Read the model definition and answer for the solid it produces. Units are mm, in the model's axes. Coordinates: 2 decimals unless noted, no trailing zeros. Loops run counter-clockwise (first coordinate to the right, second up) from the corner with the lowest first, then second, coordinate; pieces in that order, holes last.
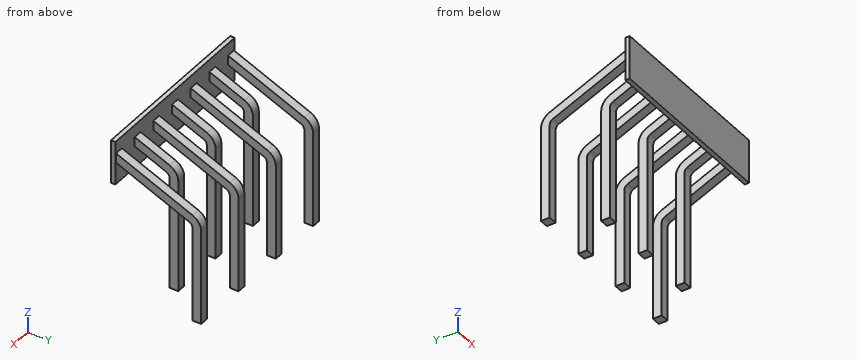
from build123d import *

# Parameters (mm, degrees)
SKETCH009_W            = 0.2
SKETCH009_H            = 2
PAD004_DEPTH           = 4.06
PAD005_DEPTH           = 0.2
LINEARPATTERN_COUNT    = 4
LINEARPATTERN_PITCH    = 2.54
PAD006_DEPTH           = 0.2
LINEARPATTERN001_COUNT = 3
LINEARPATTERN001_PITCH = 2.54


with BuildPart() as part:
    # Sketch009 (on DatumPlane) → Pad004 (new body, symmetric)
    with BuildSketch(Plane.YZ.offset(3.81)):
        with Locations((-3.8, 2.5)):
            Rectangle(SKETCH009_W, SKETCH009_H)
    extrude(amount=PAD004_DEPTH, both=True)

    # Sketch010 → Pad005 (join, symmetric)
    with BuildSketch(Plane.YZ):
        with BuildLine():
            Line((-0.2, -3.5), (-0.2, 0.85))
            ThreePointArc((-0.2, 0.85), (-0.241548, 0.988014), (-0.352383, 1.080154))
            Line((-0.352383, 1.080154), (-3.7, 2.5))
            Line((-3.7, 2.5), (-3.7, 2.934491))
            Line((-3.7, 2.934491), (-0.196196, 1.448401))
            ThreePointArc((0.2, 0.85), (0.091974, 1.208837), (-0.196196, 1.448401))
            Line((0.2, 0.85), (0.2, -3.5))
            Line((0.2, -3.5), (-0.2, -3.5))
        make_face()
    pad005 = extrude(amount=PAD005_DEPTH, both=True)

    # LinearPattern: Pad005 ×4
    with Locations(*[(i * LINEARPATTERN_PITCH, 0, 0) for i in range(1, LINEARPATTERN_COUNT)]):
        add(pad005)

    # Sketch011 (on DatumPlane) → Pad006 (join, symmetric)
    with BuildSketch(Plane.YZ.offset(1.27)):
        with BuildLine():
            Line((-3.7, 2.934491), (-3.7, 2.5))
            Line((-3.7, 2.5), (-2.257383, 1.888134))
            ThreePointArc((-2.105, 1.65798), (-2.146548, 1.795994), (-2.257383, 1.888134))
            Line((-2.105, 1.65798), (-2.105, -3.5))
            Line((-2.105, -3.5), (-1.705, -3.5))
            Line((-1.705, -3.5), (-1.705, 1.65798))
            ThreePointArc((-1.705, 1.65798), (-1.813026, 2.016816), (-2.101196, 2.256381))
            Line((-2.101196, 2.256381), (-3.7, 2.934491))
        make_face()
    pad006 = extrude(amount=PAD006_DEPTH, both=True)

    # LinearPattern001: Pad006 ×3
    with Locations(*[(i * LINEARPATTERN001_PITCH, 0, 0) for i in range(1, LINEARPATTERN001_COUNT)]):
        add(pad006)


solid = part.part
Q1. Flat-ended cylindrical pins translate along their axes: pin 1 Ø1 at (y, z) = (-2.5, 0) entering from +X; pin 2 Ø1.5 at (y, z) = (-2, 2.5) entering from -X; pin 3 Ø1.5 at (x, y) = (5.5, -3) entering from -Z. Find the tip coordinate at first contact, or state that the pin passes through.
Findings below:
pin 1: stops at x = 6.55
pin 2: stops at x = -0.2
pin 3: stops at z = 1.5
Q2. Straight lines are drawn through the part: probe 1 along X at (y, z) = (-2.05, -2.5); probe 2 along X at (y, z) = (0.05, -2.75); probe 3 along Y at (x, z) = (3.75, -0.75) (3 decimals). For each, find the intervals that lie inside material, in ascending order.
Findings below:
probe 1: x = 1.07 to 1.47, 3.61 to 4.01, 6.15 to 6.55
probe 2: x = -0.2 to 0.2, 2.34 to 2.74, 4.88 to 5.28, 7.42 to 7.82
probe 3: y = -2.105 to -1.705
Q3. A cutting plane is placed at D-D (y = -3.55). Give the vertices of the cut face in (x, z), then the cut area to 3 significant figures.
Findings below:
outline: (-0.2, 2.44) - (0.2, 2.44) - (0.2, 2.87) - (-0.2, 2.87) - close; (1.07, 2.44) - (1.47, 2.44) - (1.47, 2.87) - (1.07, 2.87) - close; (2.34, 2.44) - (2.74, 2.44) - (2.74, 2.87) - (2.34, 2.87) - close; (3.61, 2.44) - (4.01, 2.44) - (4.01, 2.87) - (3.61, 2.87) - close; (4.88, 2.44) - (5.28, 2.44) - (5.28, 2.87) - (4.88, 2.87) - close; (6.15, 2.44) - (6.55, 2.44) - (6.55, 2.87) - (6.15, 2.87) - close; (7.42, 2.44) - (7.82, 2.44) - (7.82, 2.87) - (7.42, 2.87) - close
area: 1.22 mm2
Q4. A cutting plane is placed at C-C (y = -0.1). Give the vertices of the cut face in (x, z), then the cut area to 3 significant figures.
Findings below:
outline: (-0.2, -3.5) - (0.2, -3.5) - (0.2, 1.4) - (-0.2, 1.4) - close; (2.34, -3.5) - (2.74, -3.5) - (2.74, 1.4) - (2.34, 1.4) - close; (4.88, -3.5) - (5.28, -3.5) - (5.28, 1.4) - (4.88, 1.4) - close; (7.42, -3.5) - (7.82, -3.5) - (7.82, 1.4) - (7.42, 1.4) - close
area: 7.84 mm2
Q5. A cutting plane is placed at A-A (z = -2.75). Give the vertices of the cut face in (x, y) (3 decimals).
Findings below:
outline: (-0.2, -0.2) - (0.2, -0.2) - (0.2, 0.2) - (-0.2, 0.2) - close; (1.07, -2.105) - (1.47, -2.105) - (1.47, -1.705) - (1.07, -1.705) - close; (2.34, -0.2) - (2.74, -0.2) - (2.74, 0.2) - (2.34, 0.2) - close; (3.61, -2.105) - (4.01, -2.105) - (4.01, -1.705) - (3.61, -1.705) - close; (4.88, -0.2) - (5.28, -0.2) - (5.28, 0.2) - (4.88, 0.2) - close; (6.15, -2.105) - (6.55, -2.105) - (6.55, -1.705) - (6.15, -1.705) - close; (7.42, -0.2) - (7.82, -0.2) - (7.82, 0.2) - (7.42, 0.2) - close
